```python
from build123d import *

# Parameters (mm, degrees)
BOSS_EXTRUDE4_DEPTH          = 65
SKETCH5_W                    = 73
SKETCH5_H                    = 7
SKETCH5_H_2                  = 2
BOSS_EXTRUDE5_DEPTH          = 2
CUT_EXTRUDE8_DEPTH           = 111.756489652
CUT_EXTRUDE8_DEPTH_BACK      = 5
SKETCH9_W                    = 5
SKETCH9_H                    = 3
SKETCH9_W_2                  = 2.5
BOSS_EXTRUDE8_DEPTH          = 1.5
SKETCH10_W                   = 66.5
SKETCH10_H                   = 3
BOSS_EXTRUDE9_DEPTH          = 4
M2_5X0_45_TAPPED_HOLE1_D     = 2.05
M2_5X0_45_TAPPED_HOLE1_DEPTH = 3.384117865
M2_5X0_45_TAPPED_HOLE1_TIP   = 0.615882135
SKETCH17_W                   = 11
SKETCH17_H                   = 5
BOSS_EXTRUDE20_DEPTH         = 65
CUT_EXTRUDE10_REACH          = 110.079
SKETCH18_W                   = 8
SKETCH18_H                   = 11
SKETCH20_W                   = 2.5
SKETCH20_H                   = 2
BOSS_EXTRUDE13_DEPTH         = 5.5
SKETCH22_W                   = 3.5
SKETCH22_H                   = 5
BOSS_EXTRUDE21_DEPTH         = 3
SKETCH23_W                   = 3.499642839
SKETCH23_H                   = 5
BOSS_EXTRUDE17_DEPTH         = 3
BOSS_EXTRUDE18_DEPTH         = 17.5
SKETCH27_W                   = 4
SKETCH27_H                   = 3
CUT_EXTRUDE12_DEPTH          = 5.5
M2_5X0_45_TAPPED_HOLE2_D     = 2.05
M2_5X0_45_TAPPED_HOLE2_DEPTH = 4
M2_5X0_45_TAPPED_HOLE2_TIP   = 0.615882135
SKETCH31_W                   = 8
SKETCH31_H                   = 11
SKETCH31_W_2                 = 3.2
SKETCH31_H_2                 = 8.1
BOSS_EXTRUDE22_DEPTH         = 1.5
F_5_0MM_DOWEL_HOLE1_D        = 5
F_5_0MM_DOWEL_HOLE1_DEPTH    = 5
SKETCH36_W                   = 22
SKETCH36_H                   = 89
BOSS_EXTRUDE23_DEPTH         = 5
F_8_0MM_DOWEL_HOLE1_D        = 8
F_8_0MM_DOWEL_HOLE1_DEPTH    = 2.5
F_8_0MM_DOWEL_HOLE1_TIP      = 2.403442476
SKETCH42_W                   = 2
SKETCH42_H                   = 73
BOSS_EXTRUDE25_DEPTH         = 1.5
SKETCH43_W                   = 2
SKETCH43_H                   = 73
CUT_EXTRUDE13_DEPTH          = 1.5
SKETCH44_W                   = 4
SKETCH44_H                   = 79
CUT_EXTRUDE14_DEPTH          = 1.5
SKETCH46_W                   = 5
SKETCH46_H                   = 89
BOSS_EXTRUDE26_DEPTH         = 10
SKETCH46_3_W                 = 5
SKETCH46_3_H                 = 89
BOSS_EXTRUDE27_DEPTH         = 5
FILLET1_R                    = 3
SKETCH47_W                   = 5
SKETCH47_H                   = 89
CUT_EXTRUDE15_DEPTH          = 0.1
SKETCH48_W                   = 89
SKETCH48_H                   = 4.9
CUT_EXTRUDE16_DEPTH          = 0.1


with BuildPart() as part:
    # Sketch4 → Boss-Extrude4 (new body)
    with BuildSketch(Plane(origin=(0, 0, 0), x_dir=(1, 0, 0), z_dir=(0, 1, 0))):
        Polygon((0, 0), (9, 0), (9, 89), (0, 89), (-2, 89), (-2, 81), (0, 81), (0, 84), (4, 84), (4, 5), (0, 5), (0, 8), (-2, 8), (-2, 0), align=None)
    extrude(amount=-BOSS_EXTRUDE4_DEPTH)

    # Sketch5 → Boss-Extrude5 (add)
    with BuildSketch(Plane.ZY.offset(2)):
        with Locations((-44.5, -3.5)):
            Rectangle(SKETCH5_W, SKETCH5_H)
        with Locations((-44.5, -64)):
            Rectangle(SKETCH5_W, SKETCH5_H_2)
    extrude(amount=-BOSS_EXTRUDE5_DEPTH)

    # Sketch8 → Cut-Extrude8 (cut, two sides: drawn at the far end of the back side and taken through both)
    with BuildSketch(Plane(origin=(9, 0, 0), x_dir=(0, 0, -1), z_dir=(1, 0, 0)).offset(-CUT_EXTRUDE8_DEPTH_BACK)):
        Polygon((28, 198.138247042), (28, 0), (28, -2), (68, -2), (68, 0), (68, 198.138247042), (68, 594.414741126), (28, 594.414741126), align=None)
    extrude(amount=CUT_EXTRUDE8_DEPTH + CUT_EXTRUDE8_DEPTH_BACK, mode=Mode.SUBTRACT)

    # Sketch9 → Boss-Extrude8 (add)
    with BuildSketch(Plane(origin=(9, 0, 0), x_dir=(0, 0, -1), z_dir=(1, 0, 0))):
        with Locations((86.5, -63.5)):
            Rectangle(SKETCH9_W, SKETCH9_H)
        with Locations((23.75, -63.5)):
            Rectangle(SKETCH9_W_2, SKETCH9_H)
    extrude(amount=BOSS_EXTRUDE8_DEPTH)

    # Sketch10 → Boss-Extrude9 (add)
    with BuildSketch(Plane(origin=(10.5, 0, 0), x_dir=(0, 0, -1), z_dir=(1, 0, 0))):
        with Locations((55.75, -63.5)):
            Rectangle(SKETCH10_W, SKETCH10_H)
    extrude(amount=BOSS_EXTRUDE9_DEPTH)

    # M2.5x0.45 Tapped Hole1
    with Locations(Plane(origin=(9, 0, 0), x_dir=(0, 0, -1), z_dir=(1, 0, 0))):
        with Locations((81, -5), (65.75, -19), (81, -19), (65.75, -5)):
            Hole(M2_5X0_45_TAPPED_HOLE1_D / 2, depth=M2_5X0_45_TAPPED_HOLE1_DEPTH)
            with Locations((0, 0, -(M2_5X0_45_TAPPED_HOLE1_DEPTH + M2_5X0_45_TAPPED_HOLE1_TIP / 2))):  # 118° drill point
                Cone(0, M2_5X0_45_TAPPED_HOLE1_D / 2, M2_5X0_45_TAPPED_HOLE1_TIP, mode=Mode.SUBTRACT)

    # Sketch17 → Boss-Extrude20 (add)
    with BuildSketch(Plane(origin=(0, 0, 0), x_dir=(1, 0, 0), z_dir=(0, 1, 0))):
        with Locations((14.5, 86.5)):
            Rectangle(SKETCH17_W, SKETCH17_H)
        with Locations((14.5, 2.5)):
            Rectangle(SKETCH17_W, SKETCH17_H)
    extrude(amount=-BOSS_EXTRUDE20_DEPTH)

    # Sketch18 → Cut-Extrude10 (cut, up to next)
    with BuildSketch(Plane.XY.offset(-84), mode=Mode.PRIVATE) as cut_extrude10_sk1:
        with Locations((12, -12)):
            Rectangle(SKETCH18_W, SKETCH18_H)
    cut_extrude10_tool1 = extrude(cut_extrude10_sk1.sketch, amount=-CUT_EXTRUDE10_REACH, mode=Mode.PRIVATE) & part.part
    add(cut_extrude10_tool1.solids().sort_by_distance((12, -12, -84))[0], mode=Mode.SUBTRACT)

    # Sketch20 → Boss-Extrude13 (add)
    with BuildSketch(Plane(origin=(9, 0, 0), x_dir=(0, 0, -1), z_dir=(1, 0, 0))):
        with Locations((23.75, -61)):
            Rectangle(SKETCH20_W, SKETCH20_H)
    extrude(amount=BOSS_EXTRUDE13_DEPTH)

    # Sketch22 → Boss-Extrude21 (add)
    with BuildSketch(Plane.XY.offset(-22.5)):
        with Locations((12.75, -62.5)):
            Rectangle(SKETCH22_W, SKETCH22_H)
    extrude(amount=BOSS_EXTRUDE21_DEPTH)

    # Sketch23 → Boss-Extrude17 (add)
    with BuildSketch(Plane(origin=(0, 0, -5), x_dir=(-1, 0, 0), z_dir=(0, 0, -1))):
        with Locations((-12.74982142, -62.5)):
            Rectangle(SKETCH23_W, SKETCH23_H)
    extrude(amount=BOSS_EXTRUDE17_DEPTH)

    # Sketch24 → Boss-Extrude18 (add)
    with BuildSketch(Plane(origin=(0, 0, -5), x_dir=(-1, 0, 0), z_dir=(0, 0, -1))):
        Polygon((-9, -25), (-10.6, -28), (-9, -28), align=None)
    extrude(amount=BOSS_EXTRUDE18_DEPTH)

    # Sketch25 → M1.6x0.35 Tapped Hole2 (revolve, cut)
    with BuildSketch(Plane(origin=(9, -63, -36), x_dir=(0, 0, -1), z_dir=(0, 1, 0))):
        Polygon((0, 0), (0, 4.375537887), (0.625, 4), (0.625, 0), align=None)
    revolve(axis=Axis((15.35, -63, -36), (-1, 0, 0)), mode=Mode.SUBTRACT)

    # Sketch27 → Cut-Extrude12 (cut)
    with BuildSketch(Plane(origin=(14.5, 0, 0), x_dir=(0, 0, -1), z_dir=(1, 0, 0))):
        with Locations((36, -63.5)):
            Rectangle(SKETCH27_W, SKETCH27_H)
    extrude(amount=-CUT_EXTRUDE12_DEPTH, mode=Mode.SUBTRACT)

    # M2.5x0.45 Tapped Hole2
    with Locations(Plane(origin=(6.5, 0, -4), x_dir=(0, 0, 1), z_dir=(0, 1, 0))):
        with Locations((0, 0), (-81, 0)):
            Hole(M2_5X0_45_TAPPED_HOLE2_D / 2, depth=M2_5X0_45_TAPPED_HOLE2_DEPTH)
            with Locations((0, 0, -(M2_5X0_45_TAPPED_HOLE2_DEPTH + M2_5X0_45_TAPPED_HOLE2_TIP / 2))):  # 118° drill point
                Cone(0, M2_5X0_45_TAPPED_HOLE2_D / 2, M2_5X0_45_TAPPED_HOLE2_TIP, mode=Mode.SUBTRACT)

    # Sketch31 → Boss-Extrude22 (add)
    with BuildSketch(Plane(origin=(0, 0, -84), x_dir=(-1, 0, 0), z_dir=(0, 0, -1))):
        with Locations((-12, -12)):
            Rectangle(SKETCH31_W, SKETCH31_H)
        with Locations((-12, -12)):
            Rectangle(SKETCH31_W_2, SKETCH31_H_2, mode=Mode.SUBTRACT)
    extrude(amount=BOSS_EXTRUDE22_DEPTH)

    # Ø5.0mm Dowel Hole1
    with Locations(Plane(origin=(0, 0, -5), x_dir=(-1, 0, 0), z_dir=(0, 0, -1))):
        with Locations((-12, -10)):
            Hole(F_5_0MM_DOWEL_HOLE1_D / 2, depth=F_5_0MM_DOWEL_HOLE1_DEPTH)

    # Sketch36 → Boss-Extrude23 (add)
    with BuildSketch(Plane.XZ.offset(65)):
        with Locations((9, -44.5)):
            Rectangle(SKETCH36_W, SKETCH36_H)
    extrude(amount=BOSS_EXTRUDE23_DEPTH)

    # Ø8.0mm Dowel Hole1
    with Locations(Plane.XY):
        with Locations((12, -10)):
            Hole(F_8_0MM_DOWEL_HOLE1_D / 2, depth=F_8_0MM_DOWEL_HOLE1_DEPTH)
            with Locations((0, 0, -(F_8_0MM_DOWEL_HOLE1_DEPTH + F_8_0MM_DOWEL_HOLE1_TIP / 2))):  # 118° drill point
                Cone(0, F_8_0MM_DOWEL_HOLE1_D / 2, F_8_0MM_DOWEL_HOLE1_TIP, mode=Mode.SUBTRACT)

    # Sketch42 → Boss-Extrude25 (add)
    with BuildSketch(Plane.XZ.offset(7)):
        with Locations((-1, -44.5)):
            Rectangle(SKETCH42_W, SKETCH42_H)
    extrude(amount=BOSS_EXTRUDE25_DEPTH)

    # Sketch43 → Cut-Extrude13 (cut)
    with BuildSketch(Plane(origin=(0, -63, 0), x_dir=(1, 0, 0), z_dir=(0, 1, 0))):
        with Locations((-1, 44.5)):
            Rectangle(SKETCH43_W, SKETCH43_H)
    extrude(amount=-CUT_EXTRUDE13_DEPTH, mode=Mode.SUBTRACT)

    # Sketch44 → Cut-Extrude14 (cut)
    with BuildSketch(Plane(origin=(0, -65, 0), x_dir=(1, 0, 0), z_dir=(0, 1, 0))):
        with Locations((2, 44.5)):
            Rectangle(SKETCH44_W, SKETCH44_H)
    extrude(amount=-CUT_EXTRUDE14_DEPTH, mode=Mode.SUBTRACT)



with BuildPart() as body_2:
    # Sketch46 → Boss-Extrude26 (new body)
    with BuildSketch(Plane.XZ.offset(70)):
        with Locations((27.5, -44.5)):
            Rectangle(SKETCH46_W, SKETCH46_H)
    extrude(amount=-BOSS_EXTRUDE26_DEPTH)


with BuildPart() as part_1:
    add(part.part)

    add(body_2.part)  # Boss-Extrude27 merges body 2
    # Sketch46<3> → Boss-Extrude27 (add)
    with BuildSketch(Plane.XZ.offset(70)):
        with Locations((22.5, -44.5)):
            Rectangle(SKETCH46_3_W, SKETCH46_3_H)
    extrude(amount=-BOSS_EXTRUDE27_DEPTH)

    # Fillet1
    fillet1_edges = [part_1.edges().sort_by_distance(p)[0] for p in [
        (-2, -35, 0),
        (-2, -35, -89),
        (-2, -70, -44.5),
        (14, -70, -89),
        (14, -70, 0),
    ]]
    fillet(fillet1_edges, radius=FILLET1_R)

    # Sketch47 → Cut-Extrude15 (cut)
    with BuildSketch(Plane(origin=(0, -60, 0), x_dir=(1, 0, 0), z_dir=(0, 1, 0))):
        with Locations((27.5, 44.5)):
            Rectangle(SKETCH47_W, SKETCH47_H)
    extrude(amount=-CUT_EXTRUDE15_DEPTH, mode=Mode.SUBTRACT)

    # Sketch48 → Cut-Extrude16 (cut)
    with BuildSketch(Plane.ZY.offset(-25)):
        with Locations((-44.5, -62.55)):
            Rectangle(SKETCH48_W, SKETCH48_H)
    extrude(amount=-CUT_EXTRUDE16_DEPTH, mode=Mode.SUBTRACT)


solid = part_1.part
```
Model file for the job. Use its own axes, mm. A direction names the side the tool comes from. Coordinates: 2 decimals unless noted, no trailing zeros. Order: outer loops, then holes, each group sorted by start corner. A loop starts at its lowest first (then second) coordinate and runs counter-clockwise, first axis right, second up. Notation, with made-up numbers: M -32.5,-29.5 L -13.5,-29.5 A23 cw -13.5,3.5 Z; hole C 56,-29.5 d11. An arc over 180 degrees is marked long. Answer as CSV lines item,"result".
(1) Wall check: line 1 along Z through (x, y) = (8.2, -5) (3 decimals); line 2 along X through (y, z) = (-6, -7); line 3 along Z through (x, y) = (6.5, -2.65) (3 decimals). Give the ranges that are in metal, low to high.
Geometry says:
line 1,"z = -89 to -82.025, -79.975 to -66.775, -64.725 to 0"
line 2,"x = -2 to 0, 4 to 9"
line 3,"z = -89 to -86.025, -83.975 to -5.025, -2.975 to 0"
(2) Pull direction X, two halves, no side cores. Call faces 5 (the flat face through (10.5, -63, -29)), 6 (the cylindrical face through (-1.1, -69.14, -43.92)), 7 (the flat face through (-1, -64.5, -45)), 8 (the flat face through (10, -63, -22.5)): +X half, -X half, draft (parallel to the pull), parting line (faces both ways), or undercut.
Geometry says:
face 5,"undercut"
face 6,"-X half"
face 7,"draft"
face 8,"undercut"
(3) Flat gauge pins, fed straight in: pin 1 (3 mm diameter, centred on y = -12, z = -87.5, fed in from -X); pin 2 (5 mm diameter, centred on y = -28.5, z = -16.5, fed in from -X); pin 3 (3.5 mm diameter, centred on x = 13.5, z = -7, fed in from +Y); pin 4 (6 mm diameter, centred on x = 17, z = -79.5, fed in from +Y). Where does each tip first touch, or does it go through?
Geometry says:
pin 1,"stops at x = -2"
pin 2,"stops at x = 4"
pin 3,"stops at y = -60"
pin 4,"stops at y = -62"
(4) Band-saw the part on B-B, the plane y = -26.5. List the corners of the cut face in (x, z).
Geometry says:
outline,"M -2,-86 A3 ccw 1,-89 L 20,-89 L 20,-84 L 9,-84 L 9,-22.5 L 9.8,-22.5 L 9.8,-5 L 20,-5 L 20,0 L 1,0 A3 ccw -2,-3 L -2,-8 L 0,-8 L 0,-5 L 4,-5 L 4,-84 L 0,-84 L 0,-81 L -2,-81 Z"
(5) Band-saw the part on A-A, the plane z = -24. List the corners of the cut face in (x, y).
Geometry says:
outline,"M -2,-67 A3 ccw 1,-70 L 30,-70 L 30,-60.1 L 25.1,-60.1 L 25.1,-65 L 14.5,-65 L 14.5,-60 L 9,-60 L 9,0 L 4,0 L 4,-66.5 L 0,-66.5 L 0,-64.5 L -2,-64.5 Z; M -2,-8.5 L 0,-8.5 L 0,0 L -2,0 Z"
(6) Band-saw the part on C-C, the plane x = 21.5. List the corners of the cut face in (y, z), then the cut area to 3 significant figures.
Geometry says:
outline,"M -70,-86 A3 ccw -67,-89 L -65,-89 L -65,0 L -67,0 A3 ccw -70,-3 Z"
area,"441 mm2"
(7) Band-saw the part on D-D, the plane y = -59. List the corners of the cut face in (x, z), then the cut area to 3 significant figures.
Geometry says:
outline,"M -2,-86 A3 ccw 1,-89 L 20,-89 L 20,-84 L 9,-84 L 9,-5 L 20,-5 L 20,0 L 1,0 A3 ccw -2,-3 L -2,-8 L 0,-8 L 0,-5 L 4,-5 L 4,-84 L 0,-84 L 0,-81 L -2,-81 Z"
area,"623 mm2"
(8) 3-axis set-ups, long thin cutter, end or side, ignore diameter. For faces 1 (the flat face through (10, -12, -85.5)), 2 (the flat face through (-1, -36, -81)), 3 (the flat face through (14.5, -63, -6)), 4 (the cylindrical face through (7.284, -18.692, -80.022)): which of +Z, -Z, +X, -X, +Y, -Y reach the whole face in a straight line?
Geometry says:
face 1,"-Z"
face 2,"-X"
face 3,"+Y"
face 4,"+X"
